Check sheet for the drawn part. Datum: minimum x, y, z corner. Units: mm. A direction names the side the tool comes from. Give positions to 0.01 mm unless a question says otherwise; leave off trailing zeros. Order: outer loops, then holes, each group sorted by start corner. A loop starts at its lowest first (then second) coordinate and runs counter-clockwise, first axis right, second up. Notation, with made-up numbers: (-26.75, 18.25) - (25.25, 18.25) arc R23 cw to (25.25, 35.25) - close; hole circle Ø2 at (-18.5, -1.5). An arc over 180 degrees is marked (long way). Answer as a JSON object with one key per item and string values. Group by question number.
(1) Section check A-A (y = 4.5). Record the boundary of the cut face in (x, z), then the cut area to 3 significant figures.
(2) Section check B-B (x = 58). Record the boundary of the cut face in (y, z).
(3) Depth check by flat-ended pin: pin 1 Ø5 at (x, z) = (45, 8) entering from +Y; pin 2 Ø1.5 at (x, y) = (25.5, 4) entering from -Z; pin 3 Ø4 at (x, z) = (15.5, 5) entering from -Y. Enter the tip coordinate at first touch or a pass-through.
(4) Thickness scan on line 1 (X direction, y = 3, z = 5.75); line 2 (X direction, y = 5.25, z = 4); line 3 (Y direction, x = 12, z = 4.25). Record the ranges inside material, lowest first.
(5) Access from +Z, -Z, +X, -X, +Y, -Y to the whole of each face (thin tool, end or side, straight path). Record for the marked faces 1 and 2.
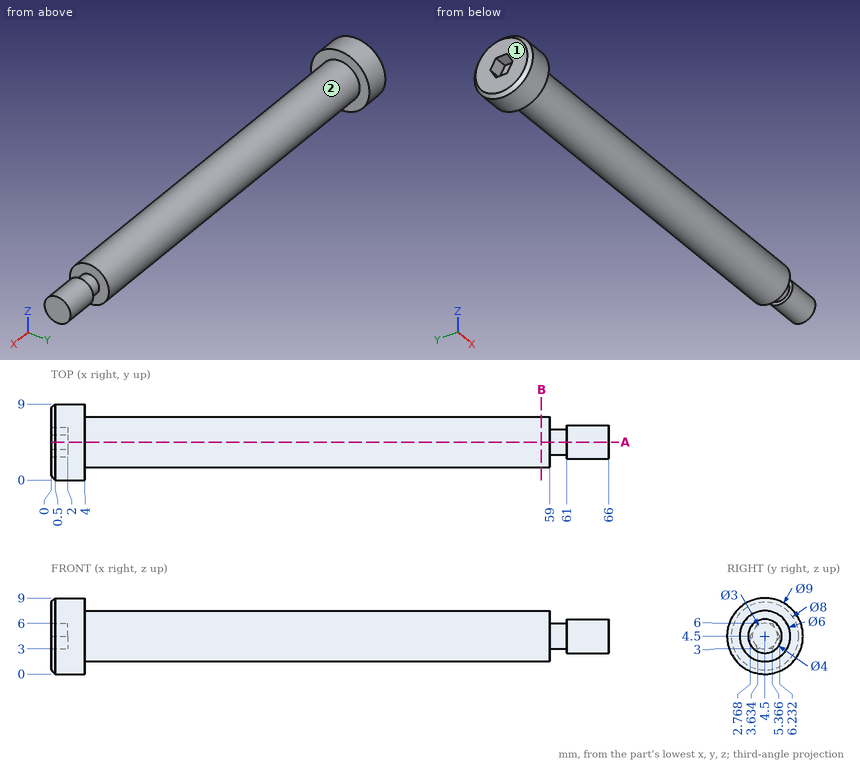
Solutions:
{
 "1": {"outline": "(0, 0.5) - (0.5, 0) - (4, 0) - (4, 1.5) - (59, 1.5) - (59, 3) - (61, 3) - (61, 2.5) - (66, 2.5) - (66, 6.5) - (61, 6.5) - (61, 6) - (59, 6) - (59, 7.5) - (4, 7.5) - (4, 9) - (0.5, 9) - (0, 8.5) - (0, 6) - (2, 6) - (2, 3) - (0, 3) - close", "area": "386 mm2"},
 "2": {"outline": "circle Ø6 at (4.5, 4.5)"},
 "3": {"pin 1": "stops at y = 7.33", "pin 2": "stops at z = 1.5", "pin 3": "stops at y = 1.5"},
 "4": {"line 1": "x = 0 to 59, 61 to 66", "line 2": "x = 2 to 66", "line 3": "y = 1.51 to 7.49"},
 "5": {"face 1": "+Z, -Z, -X, +Y, -Y", "face 2": "+X"}
}
